from build123d import *

# Parameters (mm, degrees)
SKETCH13_W          = 10
SKETCH13_H          = 10
SKETCH13_W_2        = 7
SKETCH13_H_2        = 7
BOSS_EXTRUDE1_DEPTH = 300
SKETCH15_W          = 205
SKETCH15_H          = 5
CUT_EXTRUDE1_DEPTH  = 740
SKETCH16_R          = 2.5
BOSS_EXTRUDE3_DEPTH = 50
SKETCH17_W          = 200
SKETCH17_H          = 3
CUT_EXTRUDE2_DEPTH  = 70


with BuildPart() as part:
    # Sketch13 → Boss-Extrude1 (new body)
    with BuildSketch(Plane.YZ):
        Rectangle(SKETCH13_W, SKETCH13_H)
        Rectangle(SKETCH13_W_2, SKETCH13_H_2, mode=Mode.SUBTRACT)
    extrude(amount=BOSS_EXTRUDE1_DEPTH)

    # Sketch15 → Cut-Extrude1 (cut)
    with BuildSketch(Plane(origin=(0, 5, 0), x_dir=(-1, 0, 0), z_dir=(0, 1, 0))):
        with Locations((-150, 0)):
            Rectangle(SKETCH15_W, SKETCH15_H)
    extrude(amount=-CUT_EXTRUDE1_DEPTH, mode=Mode.SUBTRACT)

    # Sketch16 → Boss-Extrude3 (add)
    with BuildSketch(Plane.XY.offset(5)):
        with Locations((5, 0)):
            Circle(SKETCH16_R)
        with Locations((295, 0)):
            Circle(SKETCH16_R)
    extrude(amount=-BOSS_EXTRUDE3_DEPTH)

    # Sketch17 → Cut-Extrude2 (cut)
    with BuildSketch(Plane.XY.offset(5)):
        with Locations((150, 0)):
            Rectangle(SKETCH17_W, SKETCH17_H)
    extrude(amount=-CUT_EXTRUDE2_DEPTH, mode=Mode.SUBTRACT)


solid = part.part
CAD build for the part. Positions are in the model's coordinates, mm. A direction names the side the tool comes from. Round coordinates to 2 decimals unless told otherwise and drop trailing zeros. Loops run counter-clockwise (first coordinate to the right, second up) from the corner with the lowest first, then second, coordinate; pieces in that order, holes last. Notation, with made-up numbers: (-15.5, -9) - (4.5, -9) arc R9 ccw to (4.5, 1) - close; hole circle Ø8 at (27.25, 15). An arc over 180 degrees is marked (long way). Put each result on its own line as item: value.
1. Pin check, flat tips, straight feed: P1, Ø5, axis at x = 87, y = -2, coming from the -Z side; P2, Ø3, axis at x = 67, z = -7.5, coming from the +Y side; P3, Ø1.5, axis at y = 3, z = -26, coming from the +X side. Stop position of each tip, or through.
Geometry check:
P1: z = -5
P2: through
P3: x = 296.09
2. 3-axis set-ups, long thin cutter, end or side, ignore diameter. For faces 1 (the flat face through (148, -2, -3.5)), 2 (the flat face through (148, -3.5, -3)), 3 (the cylindrical face through (297.31, -0.96, -24.72)), 4 (the flat face through (148, -5, -3)): which of +Z, -Z, +X, -X, +Y, -Y reach the whole face in a straight line?
Geometry check:
face 1: none
face 2: +X, -X
face 3: -Z
face 4: +Z, -Z, +X, -X, -Y
3. Slice it at C-C on x = 5. List the corners of the cut face in (y, z), and give its area (3 significant figures).
Geometry check:
outline: (-5, -5) - (-2.5, -5) - (-2.5, -45) - (2.5, -45) - (2.5, -5) - (5, -5) - (5, 5) - (-5, 5) - close; hole (-3.5, -3.5) - (-2.5, -3.5) - (-2.5, 3.5) - (-3.5, 3.5) - close; hole (2.5, -3.5) - (3.5, -3.5) - (3.5, 3.5) - (2.5, 3.5) - close
area: 286 mm²
4. Slice it at A-A on x = 199.5. List the corners of the cut face in (y, z).
Geometry check:
outline: (-5, -5) - (-1.5, -5) - (-1.5, -3.5) - (-3.5, -3.5) - (-3.5, -2.5) - (-5, -2.5) - close; (-5, 2.5) - (-3.5, 2.5) - (-3.5, 3.5) - (-1.5, 3.5) - (-1.5, 5) - (-5, 5) - close; (1.5, -5) - (5, -5) - (5, -2.5) - (3.5, -2.5) - (3.5, -3.5) - (1.5, -3.5) - close; (1.5, 3.5) - (3.5, 3.5) - (3.5, 2.5) - (5, 2.5) - (5, 5) - (1.5, 5) - close
5. Two-plate mould, pull along X, no slides. Class faces 5 (the flat face through (5, 0, -45)), 6 (the cylindrical face through (297.31, -0.96, 0.05)), 7 (the flat face through (300, -4.5, 0.1)): released by +X, released by -X, zero draft, split by the parting line, or undercut.
Geometry check:
face 5: zero draft
face 6: undercut
face 7: released by +X
6. Wall check: line 1 (Z direction, x = 45.5, y = 1.75); line 2 (Z direction, x = 252, y = 4.25). Give the ranges that are in metal, low to high.
Geometry check:
line 1: -5 to -3.5, 3.5 to 5
line 2: -5 to -2.5, 2.5 to 5
7. Slice it at D-D on z = -29. List the corners of the cut face in (x, y), and give its area (3 significant figures).
Geometry check:
outline: circle Ø5 at (5, 0); circle Ø5 at (295, 0)
area: 39.3 mm²
